Input: part model. Units: mm. Frame: model coordinates. A direction names the side the tool comes from. Coordinates: 2 decimals unless noted, no trailing zeros. Write each loop counter-clockwise with the first axis right and the second up, starting at its lowest first coordinate (ties: lowest second). Pieces come first, ordered by that corner, then holes. Notation, with made-up numbers: (41, -23.75) - (48, -23.75) arc R13 ccw to (48, -0.75) - close; hole circle Ø6 at (48, 74.5). An arc over 180 degrees is marked (long way). Use a Markdown table: item, result. Add a question column.
Q1. Section query D-D (y = -19.5). Return the cut outline in (x, z).
Q2. Section query C-C (z = 25.4). Give the number of separate pieces and of enclosed holes in the cut face, then the cut area to 3 significant figures.
Q3. Set-up query: faces 1 (the face through (135.157, 20.697, 26.831)), 2 (the face through (-2, -10, 3.099)), 3 (the face through (-120.65, 19.3, 13.3)). Return all of +Z, -Z, +X, -X, +Y, -Y with unobstructed straight access to the full face (end or side cutting, diameter ignored); none if empty.
Q4. Mould query, pull axis Y, two halves, no side actions, for faces 4 (the face through (-144.467, -2.966, 1.528)), 5 (the face through (149, 22.225, 19)), 6 (the face through (153.983, -2.966, 1.528)), 7 (the face through (149, 19.126, 20)). Classes: released by +Y, released by -Y, zero draft, split by the parting line, or undercut.
Q5. Pin query (flat end, axial travel): P1, Ø14.5, axis at x = 6.5, y = 0, coming from the +Z side; P2, Ø8.5, axis at x = 149.225, y = -3.175, coming from the +Z side; P3, Ø10.5, axis at x = 144, z = 15, coming from the -Y side; P4, Ø3.5, axis at x = -2, z = 2, coming from the +Y side. Return the tip coordinate at first contact, or that it passes through.
Q6. Section query A-A (y = 8). Return the cut outline in (x, z).
Q7. Material intervals for probe 1 along X at (y, z) = (21, 25); probe 2 along Z at (x, y) = (139.7, 20.95); probe 3 along Z at (x, y) = (-139, 21), sorted ascending. Write a range as from..to.
Q8. Section query B-B (x = 139.7). Return the cut outline in (y, z) (1 decimal), then the cut area to 3 significant figures.
from build123d import *

# Parameters (mm, degrees)
F1_DEPTH = 3.0988
F0_W     = 57.15
F0_H     = 3.0988
F2_DEPTH = 38.1
F5_D     = 9.525
F5_DEPTH = 12.7
F5_TIP   = 2.8615986981
F7_D     = 9.525
F7_DEPTH = 12.7
F7_TIP   = 2.8615986981


with BuildPart() as f1:
    # F0 (on Top) → F1 (new body)
    with BuildSketch(Plane.XY):
        Polygon((120.65, 0), (-120.65, 0), (-120.65, 19.1262), (-177.8, 19.1262), (-177.8, -28.575), (177.8, -28.575), (177.8, 19.1262), (120.65, 19.1262), align=None)
    extrude(amount=F1_DEPTH)

    # F0 (on Top) → F2 (join)
    with BuildSketch(Plane.XY):
        with Locations((-149.225, 20.6756)):
            Rectangle(F0_W, F0_H)
        with Locations((149.225, 20.6756)):
            Rectangle(F0_W, F0_H)
    extrude(amount=F2_DEPTH)

    # F5
    with Locations(Plane.XZ.offset(-19.1262)):
        with Locations((-139.7, 25.4), (139.7, 25.4)):
            Hole(F5_D / 2, depth=F5_DEPTH)
            with Locations((0, 0, -(F5_DEPTH + F5_TIP / 2))):  # 118° drill point
                Cone(0, F5_D / 2, F5_TIP, mode=Mode.SUBTRACT)

    # F7
    with Locations(Plane.XY.offset(3.0988)):
        with Locations((-149.225, -3.175), (149.225, -3.175)):
            Hole(F7_D / 2, depth=F7_DEPTH)
            with Locations((0, 0, -(F7_DEPTH + F7_TIP / 2))):  # 118° drill point
                Cone(0, F7_D / 2, F7_TIP, mode=Mode.SUBTRACT)


solid = f1.part
Values follow:
| question | item | result |
|---|---|---|
| 1 | outline | (-177.8, 0) - (177.8, 0) - (177.8, 3.1) - (-177.8, 3.1) - close |
| 2 | separate pieces | 4 |
| 2 | enclosed holes | 0 |
| 2 | area | 295 mm2 |
| 3 | face 1 | +Y, -Y |
| 3 | face 2 | +Z, +X, -X, -Y |
| 3 | face 3 | +Z, -Z, +Y |
| 4 | face 4 | undercut |
| 4 | face 5 | released by +Y |
| 4 | face 6 | undercut |
| 4 | face 7 | released by -Y |
| 5 | P1 | z = 3.1 |
| 5 | P2 | through |
| 5 | P3 | y = 19.13 |
| 5 | P4 | y = 0 |
| 6 | outline | (-177.8, 0) - (-120.65, 0) - (-120.65, 3.1) - (-177.8, 3.1) - close; (120.65, 0) - (177.8, 0) - (177.8, 3.1) - (120.65, 3.1) - close |
| 7 | probe 1 | -177.8..-144.45, -134.95..-120.65, 120.65..134.95, 144.45..177.8 |
| 7 | probe 2 | 0..20.64, 30.16..38.1 |
| 7 | probe 3 | 0..20.69, 30.11..38.1 |
| 8 | outline | (-28.6, 0) - (22.2, 0) - (22.2, 20.6) - (19.1, 20.6) - (19.1, 3.1) - (-28.6, 3.1) - close; (19.1, 30.2) - (22.2, 30.2) - (22.2, 38.1) - (19.1, 38.1) - close |
| 8 | area | 236 mm2 |
